Verification items for the finished model (mm, model axes). A direction names the side the tool comes from. Coordinates: 2 decimals unless noted, no trailing zeros. Loops run counter-clockwise (first coordinate to the right, second up) from the corner with the lowest first, then second, coordinate; pieces in that order, holes last. Notation, with made-up numbers: (74, 45.5) -> (88, 45.5) arc R19 cw to (88, 73.5) -> close; hole circle Ø4 at (8.5, -13.75). An arc over 180 degrees is marked (long way). Answer as a JSON object with one key per item and string values. Group by question number.
Q1. Gauge pin test, flat ends, axial feed: pin 1 Ø5 at (y, z) = (76, 103.5) entering from -X; pin 2 Ø12.5 at (x, z) = (5, 5.5) entering from -Y; pin 3 Ø7 at (y, z) = (-0.5, -115.5) entering from -X. Record the tip position at first contact, or that the pin passes through.
Q2. Scan lines: L1, parallel to X at y = -113.5, z = 59; L2, parallel to Y at x = -444.5, z = 21; L3, parallel to Z at x = 456, y = -4. Record each from-to range of solid material in increasing order.
Q3. Set-up check for faces 4 (the flat face through (529.44, 53, 115)), 5 (the flat face through (-160, -110.858, 0)), 6 (the flat face through (-160, 0, 110.858)), 7 (the flat face through (-160, 110.858, 0)): record each of +Z, -Z, +X, -X, +Y, -Y from which the full face is reachable in a straight line by a thin tool's end or side.
Q4. Release check for a two-part mould opening along Y. For faces 1 (the flat face through (-160, 0, -110.858)), 2 (the conical face through (-666.533, -80.338, 82.124)), 3 (the flat face through (639.44, -2, 2)) record: released by +Y, released by -Y, zero draft, split by the parting line, or undercut.
Q5. Cross-section at A-A on x = 11. Record the boundary of the cut face in (y, z) (3 decimals), and give its area (3 significant figures).
Q6. Cross-section at B-B on x = 459. Record the boundary of the cut face in (y, z), and give its area (3 significant figures).
```python
from build123d import *

# Parameters (mm, degrees)
CUT_EXTRUDE1_DEPTH = 1036.14
CIRPATTERN1_COUNT  = 4


with BuildPart() as part:
    # Sketch1 → Revolve1 (revolve)
    with BuildSketch(Plane.XY):
        Polygon((-670.560162424, 0), (-670.560162424, 110.857864376), (-656.418026801, 125), (529.439837576, 125), (529.439837576, 140), (639.439837576, 140), (639.439837576, 0), align=None)
    revolve(axis=Axis((-815.610544749, 0, 0), (1, 0, 0)))

    # Sketch2 → Cut-Extrude1 (cut)
    with BuildSketch(Plane.ZY.offset(670.560162424)):
        with BuildLine():
            Line((-20.915, 110.857864376), (20.915, 110.857864376))
            Line((20.915, 110.857864376), (20.915, 123.237830129))
            ThreePointArc((20.915, 123.237830129), (0, 125), (-20.915, 123.237830129))
            Line((-20.915, 123.237830129), (-20.915, 110.857864376))
        make_face()
    cut_extrude1 = extrude(amount=-CUT_EXTRUDE1_DEPTH, mode=Mode.SUBTRACT)

    # CirPattern1: Cut-Extrude1 ×4 about axis
    cirpattern1_axis = Axis((0, 0, 0), (1, 0, 0))
    for i in range(1, CIRPATTERN1_COUNT):
        add(cut_extrude1.rotate(cirpattern1_axis, i * 360 / CIRPATTERN1_COUNT), mode=Mode.SUBTRACT)


solid = part.part
```
Computed values:
{
 "1": {"pin 1": "stops at x = 529.44", "pin 2": "stops at y = -110.86", "pin 3": "stops at x = 365.58"},
 "2": {"L1": "x = 529.44 to 639.44", "L2": "y = -123.22 to 123.22", "L3": "z = -124.94 to 124.94"},
 "3": {"face 4": "-X", "face 5": "-X, -Y", "face 6": "+Z, -X", "face 7": "-X, +Y"},
 "4": {"face 1": "undercut", "face 2": "released by -Y", "face 3": "zero draft"},
 "5": {"outline": "(-123.238, -20.915) arc R125 ccw to (-20.915, -123.238) -> (-20.915, -110.858) -> (20.915, -110.858) -> (20.915, -123.238) arc R125 ccw to (123.238, -20.915) -> (110.858, -20.915) -> (110.858, 20.915) -> (123.238, 20.915) arc R125 ccw to (20.915, 123.238) -> (20.915, 110.858) -> (-20.915, 110.858) -> (-20.915, 123.238) arc R125 ccw to (-123.238, 20.915) -> (-110.858, 20.915) -> (-110.858, -20.915) -> close", "area": "46,800 mm²"},
 "6": {"outline": "circle Ø250 at (0, 0)", "area": "49,100 mm²"}
}
